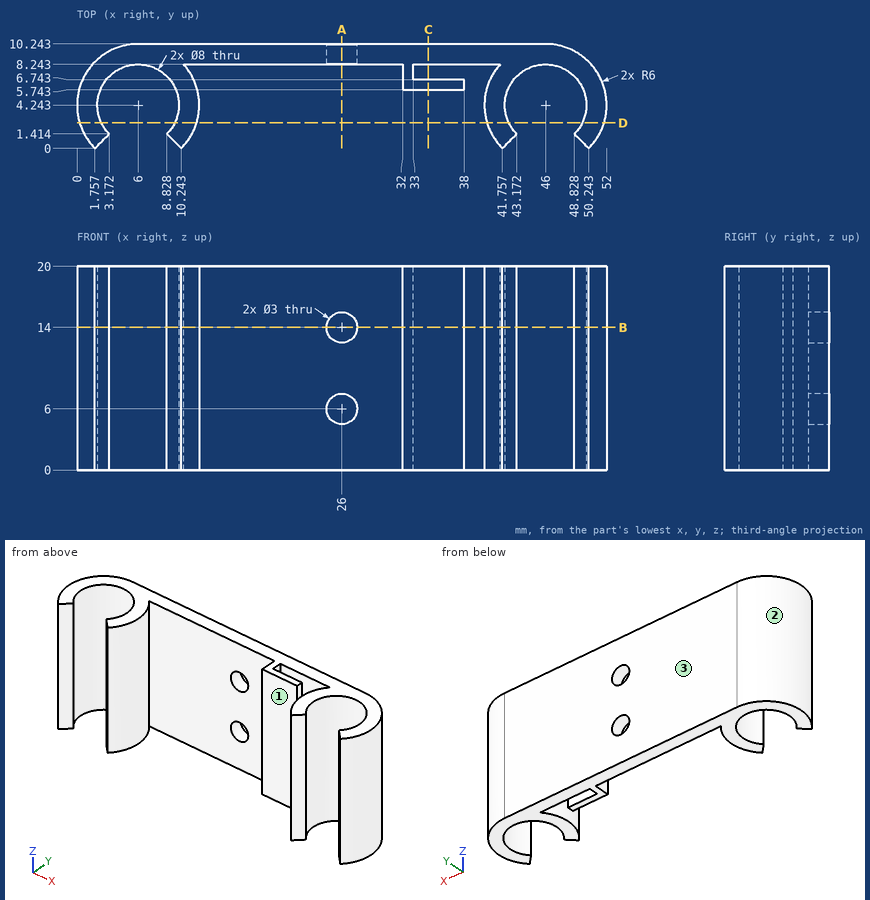
Geometry check sheet. Reference: drawing and pictorial views, mm from the part's lowest x, y, z. Give positions to 0.01 mm unless a question says otherwise; leave off trailing zeros. Order: outer loops, then holes, each group sorted by start corner. A loop starts at its lowest first (then second) coordinate and runs counter-clockwise, first axis right, second up. Notation, with made-up numbers: M 43.25,50 L 102.25,50 A18 cw 102.25,81 Z; hole C 18.25,-9.75 d8. An arc over 180 degrees is marked long. Answer as a JSON object with one key per item and string values. Group by question number.
1) Cross-section at D-D (y = 2.5). Enter the section's corners in (x, z).
2) Cross-section at A-A (x = 26). Enter the section's corners in (y, z), then the cut area to 3 significant figures.
3) Cross-section at B-B (z = 14). Enter the section's corners in (x, y) (1 decimal).
4) Scan lines: line 1 along Z through (x, y) = (26, 9.8); line 2 along X through (y, z) = (4, 16) (1 decimal); line 3 along X through (y, z) = (7, 2.75). Record each from-to range of solid material in increasing order. Write a range as [from, to].
5) Cross-section at C-C (x = 34.5). Enter the section's corners in (y, z).
6) Mould release check, pull along X, two halves, no side actions. Record for the marked faces 1, 2 and 3: released by +X, released by -X, zero draft, split by the parting line, or undercut.
7) Depth check by flat-ended pin: pin 1 Ø10 at (x, z) = (19, 11.5) entering from -Y; pin 2 Ø2.5 at (x, z) = (26, 14) entering from +Y; pin 3 Ø1 at (y, z) = (7.5, 11) entering from -X; pin 4 Ø7 at (x, z) = (35.5, 10) entering from -Y. Enter the tip coordinate at first touch or a pass-through.
Result sheet:
{
 "1": {"outline": "M 0.26,0 L 2.4,0 L 2.4,20 L 0.26,20 Z; M 9.6,0 L 11.74,0 L 11.74,20 L 9.6,20 Z; M 40.26,0 L 42.4,0 L 42.4,20 L 40.26,20 Z; M 49.6,0 L 51.74,0 L 51.74,20 L 49.6,20 Z"},
 "2": {"outline": "M 8.24,0 L 10.24,0 L 10.24,4.5 L 8.24,4.5 Z; M 8.24,7.5 L 10.24,7.5 L 10.24,12.5 L 8.24,12.5 Z; M 8.24,15.5 L 10.24,15.5 L 10.24,20 L 8.24,20 Z", "area": "28.0 mm2"},
 "3": {"outline": "M 1.8,0 L 3.2,1.4 A4 cw long 8.8,1.4 L 10.2,0 A6 ccw 10.5,8.2 L 24.5,8.2 L 24.5,10.2 L 6,10.2 A6 ccw Z; M 27.5,8.2 L 32,8.2 L 32,5.7 L 38,5.7 L 38,6.7 L 33,6.7 L 33,8.2 L 41.5,8.2 A6 ccw 41.8,0 L 43.2,1.4 A4 cw long 48.8,1.4 L 50.2,0 A6 ccw 46,10.2 L 27.5,10.2 Z"},
 "4": {"line 1": "z = [0, 4.5], [7.5, 12.5], [15.5, 20]", "line 2": "x = [0, 2], [10, 12], [40, 42], [50, 52]", "line 3": "x = [0.67, 3.1], [8.9, 11.33], [32, 33], [40.67, 43.1], [48.9, 51.33]"},
 "5": {"outline": "M 5.74,0 L 6.74,0 L 6.74,20 L 5.74,20 Z; M 8.24,0 L 10.24,0 L 10.24,20 L 8.24,20 Z"},
 "6": {"face 1": "undercut", "face 2": "released by -X", "face 3": "zero draft"},
 "7": {"pin 1": "stops at y = 8.24", "pin 2": "passes through", "pin 3": "stops at x = 0.67", "pin 4": "stops at y = 5.74"}
}
